```python
from build123d import *

# Parameters (mm, degrees)
SKETCH_1_W          = 36
SKETCH_1_H          = 16
EXTRUDE_1_DEPTH     = 1
SKETCH_2_W          = 16
SKETCH_2_H          = 37
EXTRUDE_2_DEPTH     = 1
CUT_EXTRUDE_1_REACH = 43.485
SKETCH_3_R          = 2.5
CUT_EXTRUDE_2_REACH = 54.24
SKETCH_4_R          = 2.5


with BuildPart() as part:
    # 草圖1 → 填料-伸長1 (new body)
    with BuildSketch(Plane(origin=(0, 0, 0), x_dir=(1, 0, 0), z_dir=(0, 1, 0))):
        Rectangle(SKETCH_1_W, SKETCH_1_H)
    extrude(amount=EXTRUDE_1_DEPTH)

    # 草圖2 → 填料-伸長2 (add)
    with BuildSketch(Plane(origin=(18, 0, 0), x_dir=(0, 0, -1), z_dir=(1, 0, 0))):
        with Locations((0, 18.5)):
            Rectangle(SKETCH_2_W, SKETCH_2_H)
    extrude(amount=EXTRUDE_2_DEPTH)

    # 草圖3 → 除料-伸長1 (cut, up to next)
    with BuildSketch(Plane(origin=(0, 1, 0), x_dir=(1, 0, 0), z_dir=(0, 1, 0)), mode=Mode.PRIVATE) as cut_extrude_1_sk1:
        with Locations(Location((-10, 0, 0), (0, 0, 270))):
            Circle(SKETCH_3_R)
    cut_extrude_1_tool1 = extrude(cut_extrude_1_sk1.sketch, amount=-CUT_EXTRUDE_1_REACH, mode=Mode.PRIVATE) & part.part
    # 草圖3 → 除料-伸長1 (cut, up to next)
    with BuildSketch(Plane(origin=(0, 1, 0), x_dir=(1, 0, 0), z_dir=(0, 1, 0)), mode=Mode.PRIVATE) as cut_extrude_1_sk2:
        with Locations(Location((8, 0, 0), (0, 0, 270))):
            Circle(SKETCH_3_R)
    cut_extrude_1_tool2 = extrude(cut_extrude_1_sk2.sketch, amount=-CUT_EXTRUDE_1_REACH, mode=Mode.PRIVATE) & part.part
    add(cut_extrude_1_tool1.solids().sort_by_distance((-10, 1, 0))[0], mode=Mode.SUBTRACT)
    add(cut_extrude_1_tool2.solids().sort_by_distance((8, 1, 0))[0], mode=Mode.SUBTRACT)

    # 草圖4 → 除料-伸長2 (cut, up to next)
    with BuildSketch(Plane.ZY.offset(-18), mode=Mode.PRIVATE) as cut_extrude_2_sk1:
        with Locations((0, 29)):
            Circle(SKETCH_4_R)
    cut_extrude_2_tool1 = extrude(cut_extrude_2_sk1.sketch, amount=-CUT_EXTRUDE_2_REACH, mode=Mode.PRIVATE) & part.part
    # 草圖4 → 除料-伸長2 (cut, up to next)
    with BuildSketch(Plane.ZY.offset(-18), mode=Mode.PRIVATE) as cut_extrude_2_sk2:
        with Locations((0, 11)):
            Circle(SKETCH_4_R)
    cut_extrude_2_tool2 = extrude(cut_extrude_2_sk2.sketch, amount=-CUT_EXTRUDE_2_REACH, mode=Mode.PRIVATE) & part.part
    add(cut_extrude_2_tool1.solids().sort_by_distance((18, 29, 0))[0], mode=Mode.SUBTRACT)
    add(cut_extrude_2_tool2.solids().sort_by_distance((18, 11, 0))[0], mode=Mode.SUBTRACT)


solid = part.part
```
The model under review builds one solid part; all positions refer to its coordinate system, in mm. A direction names the side the tool comes from. Round coordinates to 2 decimals unless told otherwise and drop trailing zeros. Loops run counter-clockwise (first coordinate to the right, second up) from the corner with the lowest first, then second, coordinate; pieces in that order, holes last.
Item 1: Take a section at A-A (z = 0). Write out the cut boundary in (x, y), then the cut area to 3 significant figures.
Determined:
outline: (-18, 0) - (-12.5, 0) - (-12.5, 1) - (-18, 1) - close; (-7.5, 0) - (5.5, 0) - (5.5, 1) - (-7.5, 1) - close; (10.5, 0) - (19, 0) - (19, 8.5) - (18, 8.5) - (18, 1) - (10.5, 1) - close; (18, 13.5) - (19, 13.5) - (19, 26.5) - (18, 26.5) - close; (18, 31.5) - (19, 31.5) - (19, 37) - (18, 37) - close
area: 53.0 mm2
Item 2: Mouldability with a two-part tool opening along Z and no side actions: class faces 3 (the face through (18.2, 10.2, -8)), 4 (the face through (5.56, 0.51, -0.54)), 5 (the face through (0, 0, 0)) as released by +Z, released by -Z, zero draft, split by the parting line, or undercut.
Determined:
face 3: released by -Z
face 4: undercut
face 5: zero draft
Item 3: For line 1 (X direction, y = 0.7, z = 0); line 2 (Y direction, x = 18.85, z = 0); line 3 (Y direction, x = -3, z = 1.5), list the stretches that pass through material, from the lowest coordinate up.
Determined:
line 1: x = -18 to -12.5, -7.5 to 5.5, 10.5 to 19
line 2: y = 0 to 8.5, 13.5 to 26.5, 31.5 to 37
line 3: y = 0 to 1
Item 4: Take a section at D-D (z = 6.5). Write out the cut boundary in (x, y), then the cut area to 3 significant figures.
Determined:
outline: (-18, 0) - (19, 0) - (19, 37) - (18, 37) - (18, 1) - (-18, 1) - close
area: 73.0 mm2
Item 5: For faces 1 (the face through (18.2, 10.2, 8)), 2 (the face through (18, 19, 0)), list the 3-axis set-ups (+Z, -Z, +X, -X, +Y, -Y) from which the entire face can be reached by the end or side of a thin tool; tool diameter is ignored.
Determined:
face 1: +Z, +X, -X, +Y, -Y
face 2: +Z, -Z, -X, +Y
Item 6: Take a section at C-C (y = 29). Write out the cut boundary in (x, z).
Determined:
outline: (18, -8) - (19, -8) - (19, -2.5) - (18, -2.5) - close; (18, 2.5) - (19, 2.5) - (19, 8) - (18, 8) - close
Item 7: Take a section at B-B (x = 8). Write out the cut boundary in (y, z), then the cut area to 3 significant figures.
Determined:
outline: (0, -8) - (1, -8) - (1, -2.5) - (0, -2.5) - close; (0, 2.5) - (1, 2.5) - (1, 8) - (0, 8) - close
area: 11.0 mm2
Item 8: Clearance check with flat-ended pins moving along their axes: pin 1 Ø6.5 at (y, z) = (11, 0) entering from +X; pin 2 Ø4 at (y, z) = (29, 0) entering from +X; pin 3 Ø5 at (y, z) = (20.5, 2.5) entering from -X. State where each tip first meets the part, or that it passes through.
Determined:
pin 1: stops at x = 19
pin 2: passes through
pin 3: stops at x = 18
